from build123d import *

# Parameters (mm, degrees)
SKETCH3_W           = 107
SKETCH3_H           = 25
BOSS_EXTRUDE1_DEPTH = 1.5
SKETCH3_3_W         = 1.5
SKETCH3_3_H         = 25
BOSS_EXTRUDE2_DEPTH = 25
SKETCH4_R           = 1.5
CUT_EXTRUDE1_DEPTH  = 114.495594628


with BuildPart() as part:
    # Sketch3 → Boss-Extrude1 (new body)
    with BuildSketch(Plane(origin=(0, 0, 0), x_dir=(1, 0, 0), z_dir=(0, 1, 0))):
        Rectangle(SKETCH3_W, SKETCH3_H)
    extrude(amount=-BOSS_EXTRUDE1_DEPTH)

    # Sketch3<3> → Boss-Extrude2 (add)
    with BuildSketch(Plane(origin=(0, 0, 0), x_dir=(1, 0, 0), z_dir=(0, 1, 0))):
        with Locations((-54.25, 0)):
            Rectangle(SKETCH3_3_W, SKETCH3_3_H)
        with Locations((54.25, 0)):
            Rectangle(SKETCH3_3_W, SKETCH3_3_H)
    extrude(amount=-BOSS_EXTRUDE2_DEPTH)

    # Sketch4 → Cut-Extrude1 (cut, through all)
    with BuildSketch(Plane(origin=(55, 0, 0), x_dir=(0, 0, -1), z_dir=(1, 0, 0))):
        with Locations((0, -12.5)):
            Circle(SKETCH4_R)
    extrude(amount=-CUT_EXTRUDE1_DEPTH, mode=Mode.SUBTRACT)


solid = part.part
Geometry: final body of the model. Coordinates: model frame, mm. A direction names the side the tool comes from. Coordinates: 2 decimals unless noted, no trailing zeros. Order: outer loops, then holes, each group sorted by start corner. A loop starts at its lowest first (then second) coordinate and runs counter-clockwise, first axis right, second up. Notation, with made-up numbers: M 46.5,16 L 99.5,16 A24 cw 99.5,38 Z; hole C 69,-16.5 d8. An arc over 180 degrees is marked long. One line per question, with ' | ' between items. Start each with the question number.
Item 1: Cut plane A-A, the plane z = 0. Return the cut outline in (x, y), then the cut area to 4 significant figures.
Item 2: Cut plane B-B, the plane y = -15. Return the cut outline in (x, z).
Item 3: Cut plane D-D, the plane x = -41. Return the cut outline in (y, z).
Item 4: Draft query along X for faces 3 (the cylindrical face through (54, -14, 0)), 4 (the flat face through (55, -10, 0)), 5 (the flat face through (53.5, -10, 0)), 6 (the flat face through (-1, -1.5, 0)). Return one class per face: released by +X, released by -X, zero draft, split by the parting line, or undercut.
Item 5: Cut plane C-C, the plane z = 5.25. Return the cut outline in (x, y), then the cut area to 4 significant figures.
Item 6: Set-up query: faces 1 (the flat face through (-53.5, -10, 0)), 2 (the flat face through (0, -1, 12.5)). Return all of +Z, -Z, +X, -X, +Y, -Y with unobstructed straight access to the full face (end or side cutting, diameter ignored); none if empty.
Item 7: Pin query (flat end, axial travel): pin 1 Ø12 at (x, y) = (3, -13) entering from -Z. Return the tip coordinate at first contact, or that it passes through.
Item 8: Ray query, probe 1 along X at (y, z) = (-8.25, -6); probe 2 along Y at (x, z) = (-54.65, 0); probe 3 along Y at (x, z) = (-29, -11). Return the intervals inside material, ascending. Write a range as [from, to].
A:
1) outline: M -55,-25 L -53.5,-25 L -53.5,-14 L -55,-14 Z; M -55,-11 L -53.5,-11 L -53.5,-1.5 L 53.5,-1.5 L 53.5,-11 L 55,-11 L 55,0 L -55,0 Z; M 53.5,-25 L 55,-25 L 55,-14 L 53.5,-14 Z | area: 226.5 mm2
2) outline: M -55,-12.5 L -53.5,-12.5 L -53.5,12.5 L -55,12.5 Z; M 53.5,-12.5 L 55,-12.5 L 55,12.5 L 53.5,12.5 Z
3) outline: M -1.5,-12.5 L 0,-12.5 L 0,12.5 L -1.5,12.5 Z
4) face 3: zero draft | face 4: released by +X | face 5: undercut | face 6: undercut
5) outline: M -55,-25 L -53.5,-25 L -53.5,-1.5 L 53.5,-1.5 L 53.5,-25 L 55,-25 L 55,0 L -55,0 Z | area: 235.5 mm2
6) face 1: +Z, -Z, -Y | face 2: +Z, +X, -X, +Y, -Y
7) pin 1: passes through
8) probe 1: x = [-55, -53.5], [53.5, 55] | probe 2: y = [-25, -14], [-11, 0] | probe 3: y = [-1.5, 0]
